The model under review builds one solid part; all positions refer to its coordinate system, in mm. A direction names the side the tool comes from. Round coordinates to 2 decimals unless told otherwise and drop trailing zeros. Loops run counter-clockwise (first coordinate to the right, second up) from the corner with the lowest first, then second, coordinate; pieces in that order, holes last. Notation, with made-up numbers: M 48.5,-12 L 81.5,-12 A15 ccw 81.5,5 Z; hole C 68.25,54 d11. An arc over 180 degrees is marked long. Answer as a JSON object with one key per item and string values. Group by question number.
Item 1: Consider section A-A (z = 12). Give the boundary of the cut face in (x, y).
Item 2: Tool access review of faces 1 (the face through (-37, -6.822, 6)), 2 (the face through (-37, -4, 12.7)), 3 (the face through (-18.043, -13, 6)): name each direction out of +Z, -Z, +X, -X, +Y, -Y from which nothing blocks a thin tool from reaching the whole face with its end or side.
Item 3: Consider section C-C (x = -35.5). Give the boundary of the cut face in (y, z).
Item 4: Consider section D-D (y = -22). Give the boundary of the cut face in (x, z).
Item 5: The part is to be moulded in two halves that separate along X. For faces 4 (the face through (-20.832, -13.311, 6.439)), 5 (the face through (-57, -25.4, 18)), 6 (the face through (-56.143, -13, 22)), say which applies: +X half, -X half, draft (parallel to the pull), parting line (faces both ways), or undercut.
Item 6: Consider section B-B (y = -17.5). Give the boundary of the cut face in (x, z), and give its area (3 significant figures).
Item 7: Insertion check: P1, Ø5, axis at y = -7.5, z = 21, coming from the +X side; P2, Ø1.5, axis at x = -25.5, y = -19, coming from the +Z side; P3, Ø3, axis at y = -13, z = 36, coming from the +X side; P4, Ø7.5, axis at x = -68.9, z = 33.85, coming from the +Y side. Each pin has a flat end and moves straight along its axis. Give the tip position at first contact, or say it passes through.
Item 8: To check wall thickness, follow line 1 (Y direction, x = -29, z = 3); line 2 (X direction, y = -5.5, z = 13); line 3 (Z direction, x = -55.5, y = -9.75). State the ranges of each line that lie inside material, in increasing order.
```python
from build123d import *

# Parameters (mm, degrees)
F1_DEPTH = 25.4
F2_R     = 6.35
F3_DEPTH = 25.401
F4_W     = 19.05
F4_H     = 12.7
F5_DEPTH = 12.701
F7_DEPTH = 12.701
F9_DEPTH = 12.701


with BuildPart() as f1:
    # F0 (on Front) → F1 (new body)
    with BuildSketch(Plane.XZ):
        with BuildLine():
            ThreePointArc((-56.1432969581, 31.75), (-68.5042506108, 44.4547800567), (-81.5432969581, 32.4469541982))
            Line((-81.5432969581, 32.4469541982), (-81.5432969581, 0))
            Line((-81.5432969581, 0), (-18.0432969581, 0))
            Line((-18.0432969581, 0), (-18.0432969581, 12.7))
            Line((-18.0432969581, 12.7), (-56.1432969581, 12.7))
            Line((-56.1432969581, 12.7), (-56.1432969581, 31.75))
        make_face()
    extrude(amount=F1_DEPTH)

    # F2 (on face) → F3 (cut, through all)
    with BuildSketch(Plane.XZ.offset(25.4)):
        with Locations((-68.8975006342, 33.8503867388)):
            Circle(F2_R)
    extrude(amount=-F3_DEPTH, mode=Mode.SUBTRACT)

    # F4 (on face) → F5 (cut, through all)
    with BuildSketch(Plane.XY.offset(12.7)):
        with Locations((-36.7056755349, -13.1718035824)):
            Rectangle(F4_W, F4_H)
    extrude(amount=-F5_DEPTH, mode=Mode.SUBTRACT)

    # F6 (on face) → F7 (cut, through all)
    with BuildSketch(Plane.XY.offset(12.7)):
        with BuildLine():
            Line((-46.2306755349, -19.5218035824), (-46.2306755349, -6.8218035824))
            ThreePointArc((-46.2306755349, -6.8218035824), (-52.5806755349, -13.1718035824), (-46.2306755349, -19.5218035824))
        make_face()
    extrude(amount=-F7_DEPTH, mode=Mode.SUBTRACT)

    # F8 (on face) → F9 (cut, through all)
    with BuildSketch(Plane.XY.offset(12.7)):
        with BuildLine():
            Line((-27.1806755349, -6.8218035824), (-27.1806755349, -19.5218035824))
            ThreePointArc((-27.1806755349, -19.5218035824), (-20.8306755349, -13.1718035824), (-27.1806755349, -6.8218035824))
        make_face()
    extrude(amount=-F9_DEPTH, mode=Mode.SUBTRACT)


solid = f1.part
```
Geometry results:
{
 "1": {"outline": "M -81.54,-25.4 L -18.04,-25.4 L -18.04,0 L -81.54,0 Z; hole M -46.23,-19.52 L -27.18,-19.52 A6.35 ccw -27.18,-6.82 L -46.23,-6.82 A6.35 ccw Z"},
 "2": {"face 1": "+Z, -Z", "face 2": "+Z, +X, +Y, -Y", "face 3": "+Z, -Z, +X, +Y, -Y"},
 "3": {"outline": "M -25.4,0 L -19.52,0 L -19.52,12.7 L -25.4,12.7 Z; M -6.82,0 L 0,0 L 0,12.7 L -6.82,12.7 Z"},
 "4": {"outline": "M -81.54,0 L -18.04,0 L -18.04,12.7 L -56.14,12.7 L -56.14,31.75 A12.71 ccw -81.54,32.45 Z; hole C -68.9,33.85 d12.7"},
 "5": {"face 4": "undercut", "face 5": "draft", "face 6": "+X half"},
 "6": {"outline": "M -81.54,0 L -50.88,0 L -50.88,12.7 L -56.14,12.7 L -56.14,31.75 A12.71 ccw -81.54,32.45 Z; M -22.53,0 L -18.04,0 L -18.04,12.7 L -22.53,12.7 Z; hole C -68.9,33.85 d12.7", "area": "1,060 mm^2"},
 "7": {"P1": "stops at x = -56.14", "P2": "stops at z = 12.7", "P3": "stops at x = -56.44", "P4": "passes through"},
 "8": {"line 1": "y = -25.4 to -19.52, -6.82 to 0", "line 2": "x = -81.54 to -56.14", "line 3": "z = 0 to 12.7"}
}
